Geometry: see drawing. Coordinates: mm, zero at the bounding-box minimum. Coordinates: 2 decimals unless noted, no trailing zeros. Order: outer loops, then holes, each group sorted by start corner. A loop starts at its lowest first (then second) coordinate and runs counter-clockwise, first axis right, second up. Notation, with made-up numbers: (9, -9.5) -> (43, -9.5) arc R19 ccw to (43, -2.5) -> close; hole circle Ø9 at (37, 73.5). An arc over 180 degrees is marked (long way). One line per item, written item: value. Start each with the question number.
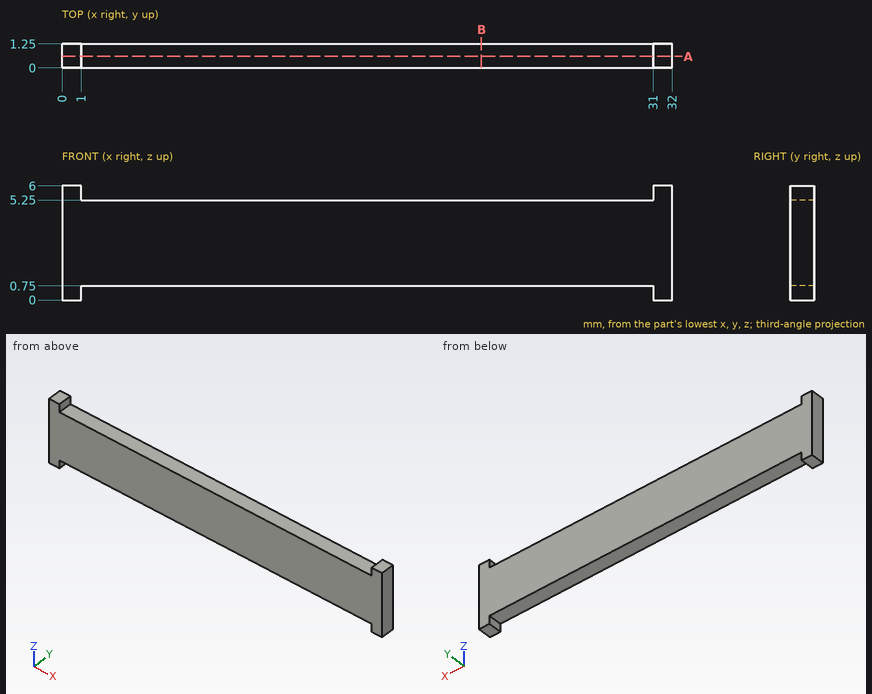
1) Ray query, line 1 along X through (y, z) = (0.3, 0.35); line 2 along Z through (x, y) = (18.5, 1). Return the intervals inside material, ascending. Write a range as from..to.
2) Section query A-A, the plane y = 0.6. Return the cut outline in (x, z).
3) Pin query (flat end, axial travel): pin 1 Ø0.6 at (x, y) = (12, 0.5) entering from -Z. Return the tip coordinate at first contact, or that it passes through.
4) Section query B-B, the plane x = 22. Return the cut outline in (y, z), plus the area to 4 significant figures.
Entries:
1. line 1: x = 0..1, 31..32
1. line 2: z = 0.75..5.25
2. outline: (0, 0) -> (1, 0) -> (1, 0.75) -> (31, 0.75) -> (31, 0) -> (32, 0) -> (32, 6) -> (31, 6) -> (31, 5.25) -> (1, 5.25) -> (1, 6) -> (0, 6) -> close
3. pin 1: stops at z = 0.75
4. outline: (0, 0.75) -> (1.25, 0.75) -> (1.25, 5.25) -> (0, 5.25) -> close
4. area: 5.625 mm2
